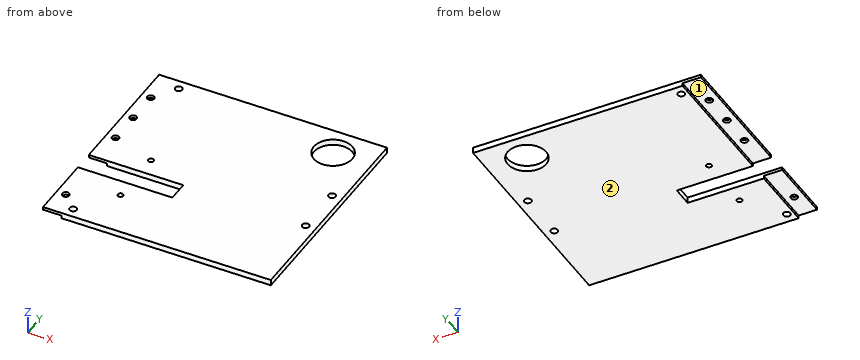
```python
from build123d import *
from OCP.BRepAlgoAPI import BRepAlgoAPI_Cut
from OCP.TopTools import TopTools_ListOfShape

# Parameters (mm, degrees)
SKETCH2_W           = 124.17
SKETCH2_H           = 119.38
BOSS_EXTRUDE1_DEPTH = 3.18
SKETCH3_R           = 1.46
SKETCH3_R_2         = 1.905
SKETCH3_R_3         = 10.5
SKETCH3_W           = 51.5
SKETCH3_H           = 11.2
CUT_EXTRUDE1_DEPTH  = 23.18
SKETCH5_W           = 1.59
SKETCH5_H           = 120
CUT_EXTRUDE2_DEPTH  = 10
SKETCH6_R           = 1.905
CUT_EXTRUDE3_DEPTH  = 10


with BuildPart() as part:
    # Sketch2 → Boss-Extrude1 (new body)
    with BuildSketch(Plane(origin=(0, -1.061487407, 0), x_dir=(1, 0, 0), z_dir=(0, 0, 1))):
        with Locations((0.708693295, -25.828343308)):
            Rectangle(SKETCH2_W, SKETCH2_H)
    extrude(amount=BOSS_EXTRUDE1_DEPTH)

    # Sketch3 → Cut-Extrude1 (cut)
    with BuildSketch(Plane.XY):
        with Locations((-32.876306705, -60.668830715)):
            Circle(SKETCH3_R)
        with Locations((-32.876306705, -29.318830715)):
            Circle(SKETCH3_R)
        with Locations((-47.826306705, 27.348169285)):
            Circle(SKETCH3_R_2)
        with Locations((41.729693295, 17.090169285)):
            Circle(SKETCH3_R_3)
        with Locations((-47.826306705, -81.127830715)):
            Circle(SKETCH3_R_2)
        with Locations((57.343693295, -13.339830715)):
            Circle(SKETCH3_R_2)
        with Locations((57.343693295, -40.439830715)):
            Circle(SKETCH3_R_2)
        with Locations((-35.626306705, -45.132830715)):
            Rectangle(SKETCH3_W, SKETCH3_H)
    extrude(amount=CUT_EXTRUDE1_DEPTH, mode=Mode.SUBTRACT)


with BuildPart() as cut_extrude2_tool:
    # Sketch5 → Cut-Extrude2 (new body)
    with BuildSketch(Plane.ZY.offset(61.376306705)):
        with Locations((0.794999799, -27.199831736)):
            Rectangle(SKETCH5_W, SKETCH5_H)
    extrude(amount=-CUT_EXTRUDE2_DEPTH)


with BuildPart() as part_1:
    add(part.part)

    # Cut-Extrude2: cut by cut_extrude2_tool, with a tolerance
    cut_extrude2_stock = TopTools_ListOfShape()
    cut_extrude2_stock.Append(part_1.part.wrapped)
    cut_extrude2_tools = TopTools_ListOfShape()
    cut_extrude2_tools.Append(cut_extrude2_tool.part.wrapped)
    cut_extrude2_cut = BRepAlgoAPI_Cut()
    cut_extrude2_cut.SetArguments(cut_extrude2_stock)
    cut_extrude2_cut.SetTools(cut_extrude2_tools)
    cut_extrude2_cut.SetFuzzyValue(0.00001)
    cut_extrude2_cut.Build()
    add(Compound.cast(cut_extrude2_cut.Shape()).solids(), mode=Mode.REPLACE)

    # Sketch6 → Cut-Extrude3 (cut)
    with BuildSketch(Plane(origin=(0, 0, 1.589999799), x_dir=(-1, 0, 0), z_dir=(0, 0, -1))):
        with Locations(Location((56.376306705, 14.720168264, 0), (0, 0, 90))):
            Circle(SKETCH6_R)
        with Locations(Location((56.376306705, -3.369831736, 0), (0, 0, 90))):
            Circle(SKETCH6_R)
        with Locations(Location((56.376306705, -21.452830715, 0), (0, 0, 90))):
            Circle(SKETCH6_R)
        with Locations(Location((56.376306705, -72.579830715, 0), (0, 0, 90))):
            Circle(SKETCH6_R)
    extrude(amount=-CUT_EXTRUDE3_DEPTH, mode=Mode.SUBTRACT)


solid = part_1.part
```
Check sheet for the modelled part. Datum: model origin and axes. Units: mm. Face numbers are marked on the shaded views. A direction names the side the tool comes from. Give positions to 0.01 mm unless a question says otherwise; leave off trailing zeros. Write each loop counter-clockwise with the first axis right and the second up, starting at its lowest first coordinate (ties: lowest second). Pieces come first, ordered by that corner, then holes. Notation, with made-up numbers: (9.5, 11) - (46.5, 11) arc R26 ccw to (46.5, 31) - close; hole circle Ø5 at (63.5, -11). An arc over 180 degrees is marked (long way). Answer as a JSON object with one key per item and string values. Group by question number.
1) Sectioned sample at B-B (y = 8.5). Record the cut outline in (x, z), then the cut area to 3 significant figures.
2) Access from +Z, -Z, +X, -X, +Y, -Y to the whole of each face (thin tool, end or side, straight path). Record for the marked faces 1 and 2.
3) Depth check by flat-ended pin: P1, Ø8, axis at x = -58.5, y = 12.5, coming from the -Z side; P2, Ø1.6, axis at y = -42.5, z = 2, coming from the -X side; P3, Ø0.5, axis at y = -74.5, z = 1, coming from the -X side. Enter the tip coordinate at first touch or a pass-through.
4) Sectioned sample at A-A (x = -37). Record the cut outline in (y, z).
5) Sectioned sample at C-C (z = 2.1). Give the number of separate pieces and of enclosed holes in the cut face, then the cut area to 3 significant figures.
6) Sectioned sample at D-D (x = 33). Record the cut outline in (y, z), then the cut area to 3 significant figures.
7) Thickness scan on probe 1 along Y at (x, z) = (-40.5, 0.6); probe 2 along X at (y, z) = (-50, 3.05); probe 3 along X at (y, z) = (17, 1.2). Record the ranges inside material, lowest first. Write a range as from..to.
Geometry results:
{
 "1": {"outline": "(-61.38, 1.59) - (-51.38, 1.59) - (-51.38, 0) - (35.69, 0) - (35.69, 3.18) - (-61.38, 3.18) - close; (47.77, 0) - (62.79, 0) - (62.79, 3.18) - (47.77, 3.18) - close", "area": "341 mm^2"},
 "2": {"face 1": "-Z, -X, +Y, -Y", "face 2": "-Z, +X, -X, +Y, -Y"},
 "3": {"P1": "stops at z = 1.59", "P2": "stops at x = -9.88", "P3": "stops at x = -51.38"},
 "4": {"outline": "(-86.58, 0) - (-50.73, 0) - (-50.73, 3.18) - (-86.58, 3.18) - close; (-39.53, 0) - (32.8, 0) - (32.8, 3.18) - (-39.53, 3.18) - close"},
 "5": {"separate pieces": "1", "enclosed holes": "11", "area": "13,800 mm^2"},
 "6": {"outline": "(-86.58, 0) - (11.26, 0) - (11.26, 3.18) - (-86.58, 3.18) - close; (22.92, 0) - (32.8, 0) - (32.8, 3.18) - (22.92, 3.18) - close", "area": "343 mm^2"},
 "7": {"probe 1": "y = -86.58..-50.73, -39.53..32.8", "probe 2": "x = -9.88..62.79", "probe 3": "x = -51.38..31.23, 52.23..62.79"}
}
